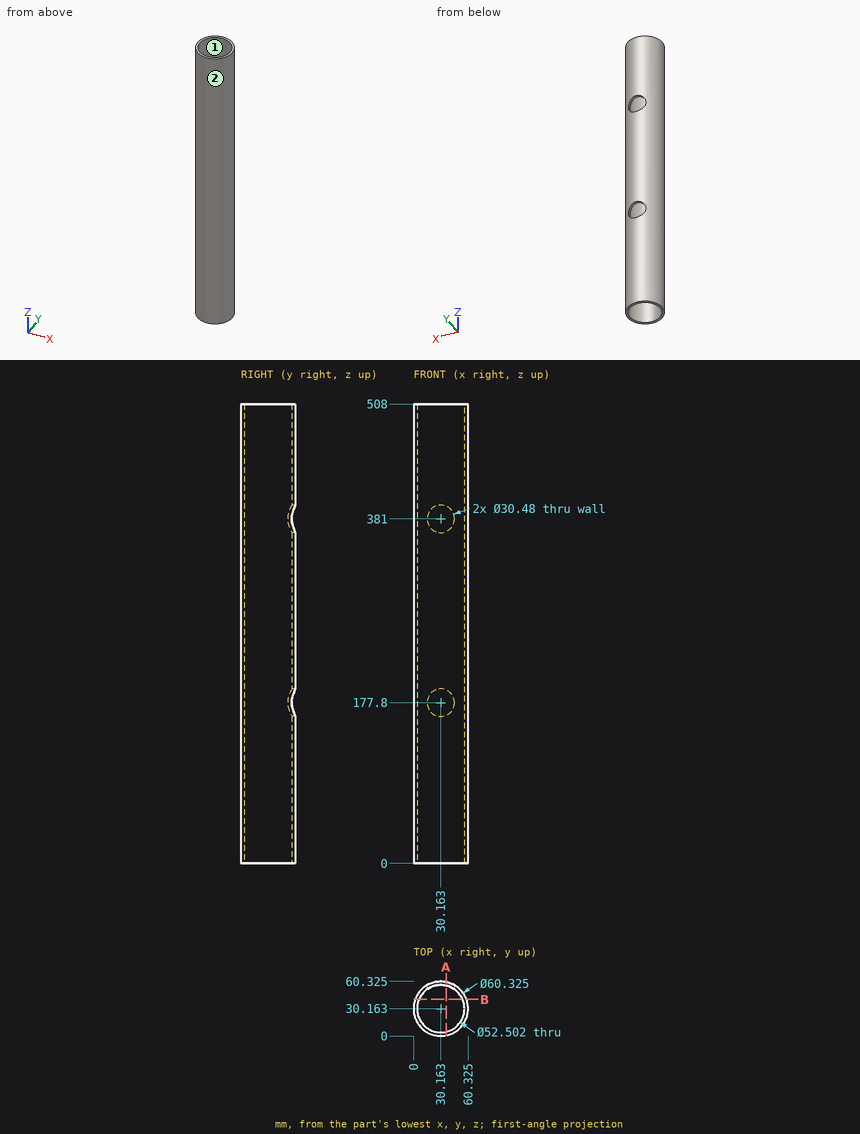
Verification items for this drawing (mm, ordinates from the low corner). Give positions to 0.01 mm unless a question says otherwise; leave off trailing zeros. Write each loop counter-clockwise with the first axis right and the second up, starting at its lowest first coordinate (ties: lowest second). Pieces come first, ordered by that corner, then holes.
1) Release check for a two-part mould opening along X. For the marked faces 1 and 2 record: pulls with the +X half, pulls with the -X half, needs draft (parallel to the pull), parting line crosses it, or undercut.
2) Section check A-A, the plane x = 36. Record the boundary of the cut face in (y, z) (1 decimal), and give its area (3 significant figures).
3) Gauge pin test, flat ends, axial feed: pin 1 (4 mm diameter, centred on y = 7.5, z = 72.5, fed in from +X) (1 decimal); pin 2 (5 mm diameter, centred on y = 36, z = 210.5, fed in from +X); pin 3 (10 mm diameter, centred on x = 52.5, z = 132.5, fed in from +Y) (1 decimal). Record the tip position at first contact, or that the pin passes through.
4) Section check B-B, the plane y = 40.5. Record the boundary of the cut face in (x, z).
5) Material ranges on L1, parallel to X at y = 29, z = 110; L2, parallel to Y at x = 31, z = 210 (1 decimal); L3, parallel to Y at x = 6, z = 363 (1 decimal), recorded low to high.
Computed:
1. face 1: undercut
1. face 2: parting line crosses it
2. outline: (0.6, 0) - (4.6, 0) - (4.6, 508) - (0.6, 508) - close; (55.8, 0) - (59.8, 0) - (59.8, 163.7) - (55.8, 163.7) - close; (55.8, 191.9) - (59.8, 191.9) - (59.8, 366.9) - (55.8, 366.9) - close; (55.8, 395.1) - (59.8, 395.1) - (59.8, 508) - (55.8, 508) - close
2. area: 3,840 mm2
3. pin 1: stops at x = 52.1
3. pin 2: stops at x = 60.14
3. pin 3: stops at y = 54.8
4. outline: (1.83, 0) - (6.03, 0) - (6.03, 508) - (1.83, 508) - close; (54.29, 0) - (58.5, 0) - (58.5, 508) - (54.29, 508) - close
5. L1: x = 0.02 to 3.94, 56.39 to 60.3
5. L2: y = 0 to 3.9, 56.4 to 60.3
5. L3: y = 12.1 to 19.9, 40.4 to 48.2
